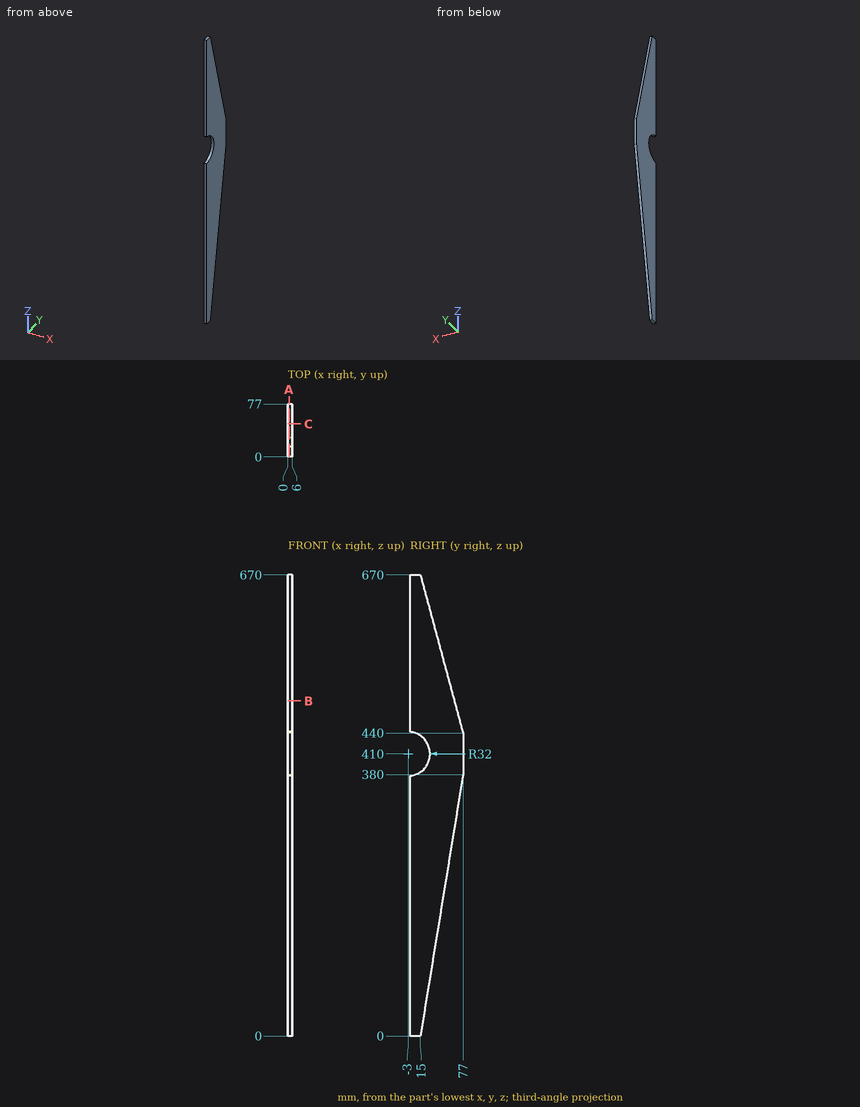
Geometry check sheet. Reference: drawing and pictorial views, mm from the part's lowest x, y, z. Round coordinates to 2 decimals unless told otherwise and drop trailing zeros. Write each loop counter-clockwise with the first axis right and the second up, starting at its lowest first coordinate (ties: lowest second). Pieces come first, ordered by that corner, then holes. Notation, with made-up numbers: (-2.75, 85.25) -> (35.25, 85.25) arc R18 cw to (35.25, 119.25) -> close; hole circle Ø5 at (-13, 25). An arc over 180 degrees is marked (long way). Put each result on its own line as item: value.
1) Depth check by flat-ended pin: P1, Ø2, axis at x = 3.5, z = 372, coming from the +Y side. Enter the tip coordinate at first touch or a pass-through.
Recorded:
P1: stops at y = 75.86
2) Cross-section at C-C, the plane y = 48. Enter the section's corners in (x, z), plus the area to 3 significant figures.
Recorded:
outline: (0, 202.26) -> (6, 202.26) -> (6, 547.58) -> (0, 547.58) -> close
area: 2,070 mm2
3) Cross-section at B-B, the plane z = 487. Enter the section's corners in (x, y).
Recorded:
outline: (0, 0) -> (6, 0) -> (6, 64.33) -> (0, 64.33) -> close
4) Cross-section at A-A, the plane x = 1.8. Enter the section's corners in (y, z), plus the area to 3 significant figures.
Recorded:
outline: (0, 0) -> (15, 0) -> (77, 380) -> (77, 440) -> (15, 670) -> (0, 670) -> (0, 441.86) arc R32 cw to (0, 378.14) -> close
area: 31,300 mm2
5) Thickness scan on probe 1 along Z at (x, y) = (0.65, 10.5); probe 2 along Y at (x, z) = (0.95, 494); probe 3 along Y at (x, z) = (2.6, 396.5). Record the ranges inside material, lowest first. Write a range as from..to.
Recorded:
probe 1: z = 0..380.99, 439.01..670
probe 2: y = 0..62.44
probe 3: y = 26.01..77
